Check sheet for the drawn part. Datum: minimum x, y, z corner. Units: mm. A direction names the side the tool comes from. Round coordinates to 2 decimals unless told otherwise and drop trailing zeros. Order: outer loops, then holes, each group sorted by start corner. A loop starts at its lowest first (then second) coordinate and runs counter-clockwise, first axis right, second up. Notation, with made-up numbers: (15, 75.25) -> (23, 75.25) arc R25 cw to (23, 112.25) -> close; hole circle Ø5 at (-10, 4). An arc over 180 degrees is marked (long way). Answer in a Markdown table with one row per item.
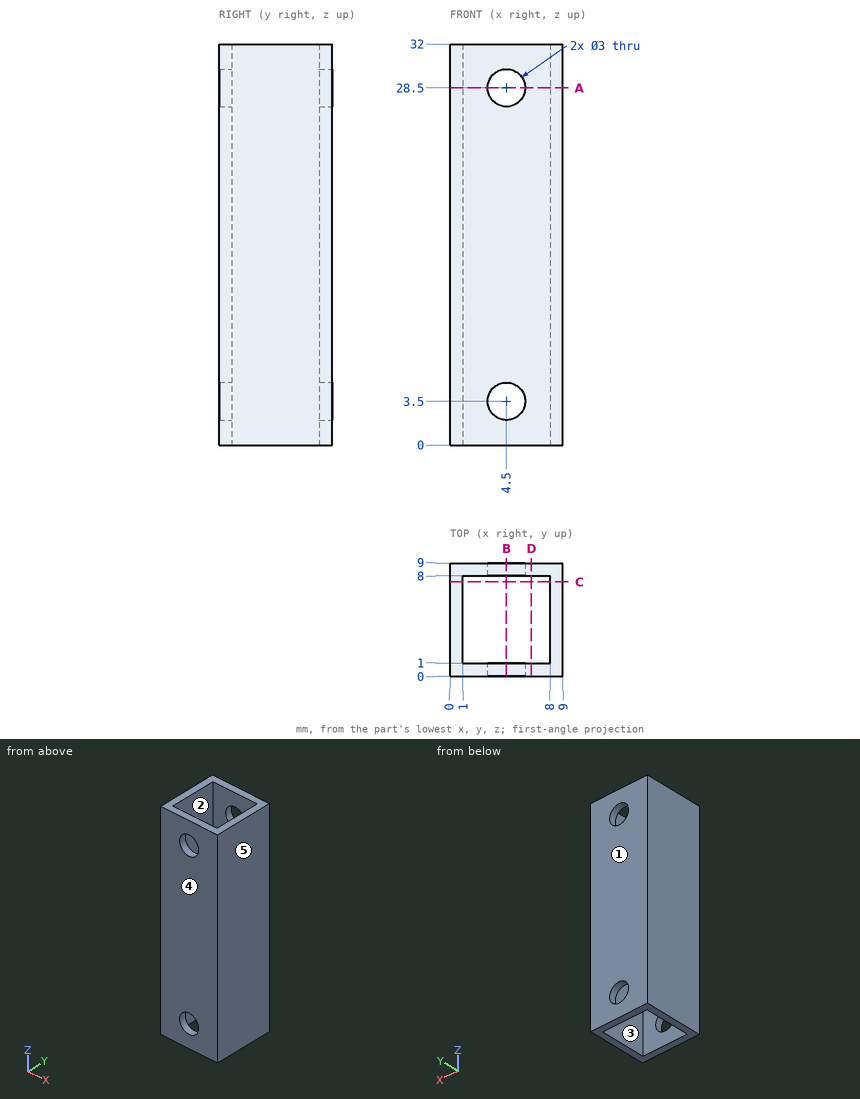
(1) Scan lines: probe 1 along Z at (x, y) = (4.5, 8.65); probe 2 along Y at (x, z) = (4.5, 21); probe 3 along X at (y, z) = (8.35, 3.5). Record each from-to range of solid material in increasing order. Write a range as from..to.
Solutions:
| item | result |
|---|---|
| probe 1 | 0..2, 5..27, 30..32 |
| probe 2 | 0..1, 8..9 |
| probe 3 | 0..3, 6..9 |
(2) Draft check along X on the marked faces 3, 4 and 5. Enter one of: pulls with the +X half, pulls with the -X half, needs draft (parallel to the pull), parting line crosses it, or undercut.
Solutions:
| item | result |
|---|---|
| face 3 | undercut |
| face 4 | needs draft |
| face 5 | pulls with the +X half |
(3) Tool access check on the marked faces 1 and 2. Record the directions out of +Z, -Z, +X, -X, +Y, -Y that give a thin tool (end or side, any length) a straight path to the whole face; none if there is none.
Solutions:
| item | result |
|---|---|
| face 1 | +Z, -Z, +X, -X, +Y |
| face 2 | +Z, -Z |
(4) Section check C-C on y = 7.5. Record the boundary of the cut face in (x, z), plus the area to 3 significant figures.
Solutions:
| item | result |
|---|---|
| outline | (0, 0) -> (1, 0) -> (1, 32) -> (0, 32) -> close; (8, 0) -> (9, 0) -> (9, 32) -> (8, 32) -> close |
| area | 64.0 mm^2 |
(5) Section check A-A on z = 28.5. Record the boundary of the cut face in (x, y), plus the area to 3 significant figures.
Solutions:
| item | result |
|---|---|
| outline | (0, 0) -> (3, 0) -> (3, 1) -> (1, 1) -> (1, 8) -> (3, 8) -> (3, 9) -> (0, 9) -> close; (6, 0) -> (9, 0) -> (9, 9) -> (6, 9) -> (6, 8) -> (8, 8) -> (8, 1) -> (6, 1) -> close |
| area | 26.0 mm^2 |
(6) Section check B-B on x = 4.5. Record the boundary of the cut face in (y, z).
Solutions:
| item | result |
|---|---|
| outline | (0, 0) -> (1, 0) -> (1, 2) -> (0, 2) -> close; (0, 5) -> (1, 5) -> (1, 27) -> (0, 27) -> close; (0, 30) -> (1, 30) -> (1, 32) -> (0, 32) -> close; (8, 0) -> (9, 0) -> (9, 2) -> (8, 2) -> close; (8, 5) -> (9, 5) -> (9, 27) -> (8, 27) -> close; (8, 30) -> (9, 30) -> (9, 32) -> (8, 32) -> close |
(7) Depth check by flat-ended pin: pin 1 Ø2.5 at (x, z) = (4.5, 3.5) entering from -Y. Enter the tip coordinate at first touch or a pass-through.
Solutions:
| item | result |
|---|---|
| pin 1 | through |
